Check sheet for the modelled part. Datum: model origin and axes. Units: mm. Face numbers are marked on the shaded views. A direction names the side the tool comes from. Round coordinates to 2 decimals unless told otherwise and drop trailing zeros. Order: outer loops, then holes, each group sorted by start corner. A loop starts at its lowest first (then second) coordinate and runs counter-clockwise, first axis right, second up. Notation, with made-up numbers: (30.5, -17) -> (44.5, -17) arc R15 cw to (44.5, 9) -> close; hole circle Ø8 at (25.25, 19). An arc over 180 degrees is marked (long way). Use CSV: the item, a comma, the result in double quotes.
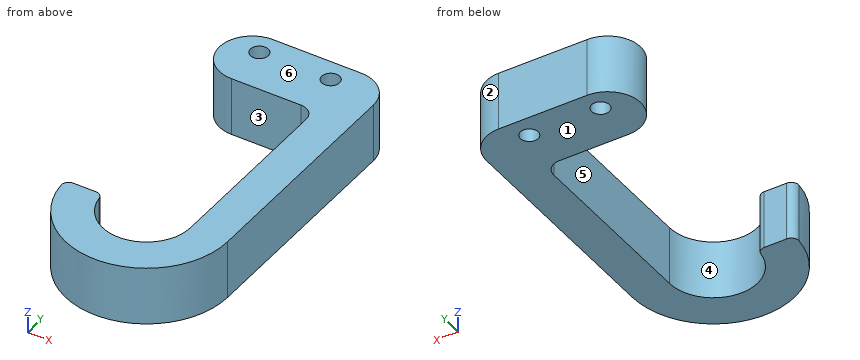
```python
from build123d import *

# Parameters (mm, degrees)
F0_R     = 1.9332973568
F1_DEPTH = 6.35


# Not quite as in the source:
# - a feature names something its author has since deleted; it is built from what else it names


with BuildPart() as f1:
    # F0 (on Top) → F1 (new body, symmetric)
    with BuildSketch(Plane.XY):
        with BuildLine():
            ThreePointArc((-15.8833512398, 0), (-17.0603794097, -0.5222484159), (-17.4629810004, -1.7453799214))
            ThreePointArc((-17.4629810004, -1.7453799214), (0.8737735944, -17.5282222771), (17.5499873644, 0))
            Line((17.5499873644, 0), (17.5499873644, 49.6334969772))
            ThreePointArc((17.5499873644, 49.6334969772), (15.4732281229, 54.6472373039), (10.4594877962, 56.7239965454))
            Line((10.4594877962, 56.7239965454), (-8.711161666, 56.7239965454))
            ThreePointArc((-8.711161666, 56.7239965454), (-14.3252844017, 53.9644102799), (-15.5694312717, 47.8336852809))
            ThreePointArc((-15.5694312717, 47.8336852809), (-13.0420749687, 44.0193742416), (-8.711161666, 42.5429974091))
            Line((-8.711161666, 42.5429974091), (6.35, 42.5429974091))
            ThreePointArc((6.35, 42.5429974091), (8.5950640303, 41.6130614393), (9.525, 39.3679974091))
            Line((9.525, 39.3679974091), (9.525, 0))
            ThreePointArc((9.525, 0), (0.6821084333, -9.5005448836), (-9.4273051098, -1.3607142857))
            ThreePointArc((-9.4273051098, -1.3607142857), (-9.9592599258, -0.3874627982), (-10.9985226281, 0))
            Line((-10.9985226281, 0), (-15.8833512398, 0))
        make_face()
        with Locations((-8.711161666, 52.084082889)):
            Circle(F0_R, mode=Mode.SUBTRACT)
        with Locations((6.7552171887, 52.084082889)):
            Circle(F0_R, mode=Mode.SUBTRACT)
    extrude(amount=F1_DEPTH, both=True)


solid = f1.part
```
Q1. Sectioned sample at D-D, the plane y = 38.5. Enter the section's corners in (x, z) (3 decimals), then the cut area to 3 significant figures.
Result sheet:
outline,"(9.525, -6.35) -> (17.55, -6.35) -> (17.55, 6.35) -> (9.525, 6.35) -> close"
area,"102 mm^2"
Q2. Go/stop test with flat-tipped pins: pin 1 (3 mm diameter, centred on x = -8.71, y = 52.08, fed in from -Z); pin 2 (2 mm diameter, centred on y = 8.5, z = 0.5, fed in from -X) (3 decimals); pin 3 (5.5 mm diameter, centred on x = -14.5, z = 2, fed in from +Y). Record where each tip stops, or that it passes through.
Result sheet:
pin 1,"passes through"
pin 2,"stops at x = 9.525"
pin 3,"stops at y = 56.04"
Q3. Scan lines: L1, parallel to Y at x = -7, z = -4.5; L2, parallel to X at y = 36.5, z = -5.5 (3 decimals); L3, parallel to Y at x = 7.5, z = 2.5. Record each from-to range of solid material in increasing order.
Result sheet:
L1,"y = -16.09 to -6.46, 42.54 to 51.18, 52.98 to 56.72"
L2,"x = 9.525 to 17.55"
L3,"y = -15.87 to -5.87, 42.33 to 50.3, 53.87 to 56.72"
Q4. Mould release check, pull along Y, two halves, no side actions. Record for the marked faces 1, 2 and 3: pulls with the +Y half, pulls with the -Y half, needs draft (parallel to the pull), parting line crosses it, or undercut.
Result sheet:
face 1,"needs draft"
face 2,"pulls with the +Y half"
face 3,"undercut"
Q5. Sectioned sample at B-B, the plane y = -7. Enter the section's corners in (x, z), then the cut area to 3 significant figures.
Result sheet:
outline,"(-16.09, -6.35) -> (-6.46, -6.35) -> (-6.46, 6.35) -> (-16.09, 6.35) -> close; (6.46, -6.35) -> (16.09, -6.35) -> (16.09, 6.35) -> (6.46, 6.35) -> close"
area,"245 mm^2"
Q6. Sectioned sample at A-A, the plane x = 0. Enter the section's corners in (y, z) (3 decimals).
Result sheet:
outline,"(-17.55, -6.35) -> (-9.525, -6.35) -> (-9.525, 6.35) -> (-17.55, 6.35) -> close; (42.543, -6.35) -> (56.724, -6.35) -> (56.724, 6.35) -> (42.543, 6.35) -> close"
Q7. Access from +Z, -Z, +X, -X, +Y, -Y to the whole of each face (thin tool, end or side, straight path). Record for the marked faces 4, 5 and 6.
Result sheet:
face 4,"+Z, -Z"
face 5,"+Z, -Z, -X"
face 6,"+Z, +X, -X, +Y, -Y"
Q8. Sectioned sample at C-C, the plane z = -5. State how many separate pieces and enclosed holes the cut face has, then the cut area to 3 significant figures.
Result sheet:
separate pieces,"1"
enclosed holes,"2"
area,"1,100 mm^2"
